Autodesk Inventor part; units mm, degrees
ref_plane "YZ Plane" through (0, 0, 0) normal (1, 0, 0) x (0, 1, 0)
ref_plane "XZ Plane" through (0, 0, 0) normal (0, 1, 0) x (-1, 0, 0)
ref_plane "XY Plane" through (0, 0, 0) normal (0, 0, 1) x (1, 0, 0)
sketch "Sketch1" plane through (0, 0, 0) normal (0, 1, 0) x (-1, 0, 0)
  line L0 (3.175, 0) -> (53.225, 0)
  line L1 (56.4, -3.175) -> (56.4, -53.225)
  line L2 (53.225, -56.4) -> (3.175, -56.4)
  line L3 (0, -53.225) -> (0, -3.175)
  arc A0 (56.4, -3.175) -> (53.225, 0) centre (53.225, -3.175) ccw
  arc A1 (3.175, 0) -> (0, -3.175) centre (3.175, -3.175) ccw
  arc A2 (0, -53.225) -> (3.175, -56.4) centre (3.175, -53.225) ccw
  arc A3 (53.225, -56.4) -> (56.4, -53.225) centre (53.225, -53.225) ccw
  point P0 (0, 0)
  point P1 (56.4, -56.4)
  point P2 (56.4, 0)
  point P3 (0, -56.4)
  dimension "d0" = 56.4
  dimension "d1" = 56.4
  dimension "d2" = 3.175
extrude "Extrusion1" add sketch "Sketch1" along normal blind 56
sketch "Sketch2" plane through (0, 56, 0) normal (0, 1, 0) x (1, 0, 0)
  line L0 (0, 0) -> (-56.4, 0) construction
  line L1 (-56.4, 0) -> (-56.4, 56.4) construction
  line L2 (-56.4, 56.4) -> (0, 56.4) construction
  line L3 (0, 56.4) -> (0, 0) construction
  line L4 (-56.4, 0) -> (0, 56.4) construction
  line L5 (-4.63, 4.63) -> (-51.77, 4.63) construction
  line L6 (-51.77, 4.63) -> (-51.77, 51.77) construction
  line L7 (-51.77, 51.77) -> (-4.63, 51.77) construction
  line L8 (-4.63, 51.77) -> (-4.63, 4.63) construction
  line L9 (-4.63, 4.63) -> (-51.77, 51.77) construction
  line L10 (-51.77, 4.63) -> (-4.63, 51.77) construction
  circle A0 centre (-51.8006, 4.5994) radius 2.5
  circle A1 centre (-51.77, 51.77) radius 2.5
  circle A2 centre (-4.63, 51.77) radius 2.5
  circle A3 centre (-4.63, 4.63) radius 2.5
  point P0 (-28.2, 28.2)
  dimension "d5" = 47.14
  dimension "d6" = 47.14
  dimension "d7" = 5
  dimension "d8" = 5
  dimension "d9" = 5
  dimension "d10" = 5
sketch "Sketch3" plane through (0, 56, 0) normal (0, 1, 0) x (1, 0, 0)
  line L0 (0, 0) -> (-56.4, 56.4) construction
  circle A0 centre (-28.2, 28.2) radius 19.05
  dimension "d18" = 38.1
extrude "Extrusion2" add sketch "Sketch3" along normal blind 1.6
sketch "Sketch4" plane through (-28.2, 57.6, -28.2) normal (0, 1, 0) x (1, 0, 0)
  circle A0 centre (0, 0) radius 3.175
  point P0 (28.2, -28.2)
  dimension "d21" = 6.35
extrude "Extrusion3" add sketch "Sketch4" along normal blind 21
extrude "Extrusion4" cut sketch "Sketch2" against normal through all
sketch "Sketch5" plane through (-53.225, 0, 0) normal (0, 0, 1) x (1, 0, 0)
  line L0 (-3.175, 0) -> (-3.175, 56) construction
  line L1 (-3.175, 56) -> (3.9116, 56) construction
  line L2 (3.9116, 56) -> (3.9116, 51) construction
  line L3 (3.9116, 51) -> (-3.175, 51) construction
  line L4 (-3.175, 51) -> (-3.175, 56) construction
  line L5 (-3.175, 51) -> (3.9116, 51)
  line L6 (3.9116, 51) -> (3.9116, 0)
  line L7 (3.9116, 0) -> (-3.175, 0)
  line L8 (-3.175, 0) -> (-3.175, 51)
  line L9 (50.05, 0) -> (0, 0) construction
  line L10 (25.025, 0) -> (25.025, 56) construction
  line L11 (50.05, 56) -> (0, 56) construction
  line L12 (53.225, 0) -> (53.225, 56) construction
  line L13 (53.225, 56) -> (46.1384, 56) construction
  line L14 (46.1384, 56) -> (46.1384, 51) construction
  line L15 (46.1384, 51) -> (53.225, 51) construction
  line L16 (53.225, 51) -> (53.225, 56) construction
  line L17 (53.225, 51) -> (46.1384, 51)
  line L18 (46.1384, 51) -> (46.1384, 0)
  line L19 (46.1384, 0) -> (53.225, 0)
  line L20 (53.225, 0) -> (53.225, 51)
  point P0 (53.225, 0)
  point P1 (55.3116, 56)
  dimension "d26" = 7.0866
  dimension "d27" = 5
extrude "Extrusion5" cut sketch "Sketch5" against normal blind 7.0866
sketch "Sketch6" plane through (-3.175, 0, -56.4) normal (0, 0, -1) x (-1, 0, 0)
  line L0 (-3.175, 0) -> (-3.175, 56) construction
  line L1 (-3.175, 56) -> (3.9116, 56) construction
  line L2 (3.9116, 56) -> (3.9116, 51) construction
  line L3 (3.9116, 51) -> (-3.175, 51) construction
  line L4 (-3.175, 51) -> (-3.175, 56) construction
  line L5 (-3.175, 51) -> (3.9116, 51)
  line L6 (3.9116, 51) -> (3.9116, 0)
  line L7 (3.9116, 0) -> (-3.175, 0)
  line L8 (-3.175, 0) -> (-3.175, 51)
  line L9 (50.05, 0) -> (0, 0) construction
  line L10 (25.025, 0) -> (25.025, 56) construction
  line L11 (50.05, 56) -> (0, 56) construction
  line L12 (53.225, 0) -> (53.225, 56) construction
  line L13 (53.225, 56) -> (46.1384, 56) construction
  line L14 (46.1384, 56) -> (46.1384, 51) construction
  line L15 (46.1384, 51) -> (53.225, 51) construction
  line L16 (53.225, 51) -> (53.225, 56) construction
  line L17 (53.225, 51) -> (46.1384, 51)
  line L18 (46.1384, 51) -> (46.1384, 0)
  line L19 (46.1384, 0) -> (53.225, 0)
  line L20 (53.225, 0) -> (53.225, 51)
  point P0 (-3.175, 0)
  point P1 (53.225, 0)
  point P2 (55.3116, 56)
  dimension "d32" = 7.0866
  dimension "d33" = 5
extrude "Extrusion6" cut sketch "Sketch6" against normal blind 7.0866
properties part number "NEMA23 Motor"
The listing builds one solid part. Answer for the finished solid, in the listing's coordinates (mm). A direction names the side the tool comes from. Coordinates: 2 decimals unless noted, no trailing zeros. Order: outer loops, then holes, each group sorted by start corner. A loop starts at its lowest first (then second) coordinate and runs counter-clockwise, first axis right, second up. Notation, with made-up numbers: M 69.25,18.5 L 73.25,18.5 A9 ccw 73.25,27.5 Z; hole C 37.5,-24 d6. An arc over 180 degrees is marked long. Answer as a JSON object with one key per item and string values. Group by question number.
1. Flat-ended cylindrical pins translate along their axes: P1, Ø6, axis at x = -21, y = 57.5, coming from the +Z side; P2, Ø2, axis at y = 59.5, z = -12.5, coming from the -X side; P3, Ø1.1, axis at x = -50.5, y = 38, coming from the +Z side; P4, Ø1.2, axis at y = 35, z = -1.5, coming from the +X side. Find the tip coordinate at first contact, or state that the pin passes through.
2. Section A-A on z = -28.2 is taken. Write down the section's boundary in (x, y) (3 decimals), then the cut area to 3 significant figures.
3. Determine the mould class of faces 1 (the flat face through (-54, 51, -3)), 2 (the cylindrical face through (-4.448, 38.501, -7.123)), 3 (the cylindrical face through (-49.283, 38.501, -52.024)), 4 (the flat face through (-50, 26, -7.087)) for opening direction Z: released by +Z, released by -Z, zero draft, split by the parting line, or undercut.
4. A tool of negligible diameter and unlimited length cuts with its end or side. For faces 5 (the flat face through (-2, 26, -7.087)), 6 (the flat face through (-49.313, 26, -6)), 7 (the flat face through (-3, 51, -54)), 8 (the flat face through (-49.313, 26, -50)), 9 (the cylindrical face through (-30.72, 67.95, -30.13)), from which of +Z, -Z, +X, -X, +Y, -Y can it reach the whole face along a straight path? Write none if from no direction.
5. Section C-C on x = -15.5 is taken. Write down the section's boundary in (y, z).
6. Straight lines are drawn through the part: line 1 (Y direction, x = -52, z = -12); line 2 (Z direction, x = -4.63, y = 18.5); line 3 (Y direction, x = -23.5, z = -32). For each, find the intervals that lie inside material, in ascending order.
7. Section B-B on y = 12.5 is taken. Write down the section's boundary in (x, z).
8. Section D-D on z = -44 is taken. Write down the section's boundary in (x, y).
Values follow:
{
 "1": {"P1": "z = 0", "P2": "through", "P3": "z = -7.09", "P4": "x = -7.09"},
 "2": {"outline": "M -56.4,0 L 0,0 L 0,56 L -9.15,56 L -9.15,57.6 L -25.025,57.6 L -25.025,78.6 L -31.375,78.6 L -31.375,57.6 L -47.25,57.6 L -47.25,56 L -56.4,56 Z", "area": "3,350 mm2"},
 "3": {"face 1": "zero draft", "face 2": "undercut", "face 3": "undercut", "face 4": "released by +Z"},
 "4": {"face 5": "+Z, +X, -Y", "face 6": "+Z, -X, -Y", "face 7": "-Z, +X, -Y", "face 8": "-Z, -X, -Y", "face 9": "+Y"},
 "5": {"outline": "M 0,-56.4 L 56,-56.4 L 56,-42.4 L 57.6,-42.4 L 57.6,-14 L 56,-14 L 56,0 L 0,0 Z"},
 "6": {"line 1": "0 to 56", "line 2": "-49.27 to -7.13", "line 3": "0 to 57.6"},
 "7": {"outline": "M -56.4,-49.31 L -52.23,-49.31 A2.5 cw -51.31,-49.31 L -49.31,-49.31 L -49.31,-51.31 A2.5 cw -49.31,-52.23 L -49.31,-56.4 L -7.09,-56.4 L -7.09,-52.23 A2.5 cw -7.09,-51.31 L -7.09,-49.31 L -5.09,-49.31 A2.5 cw -4.17,-49.31 L 0,-49.31 L 0,-7.09 L -4.17,-7.09 A2.5 cw -5.09,-7.09 L -7.09,-7.09 L -7.09,-5.09 A2.5 cw -7.09,-4.17 L -7.09,0 L -49.31,0 L -49.31,-4.35 A2.5 cw -49.31,-4.85 L -49.31,-7.09 L -51.55,-7.09 A2.5 cw -52.05,-7.09 L -56.4,-7.09 Z"},
 "8": {"outline": "M -56.4,0 L 0,0 L 0,56 L -17.56,56 L -17.56,57.6 L -38.84,57.6 L -38.84,56 L -56.4,56 Z"}
}
